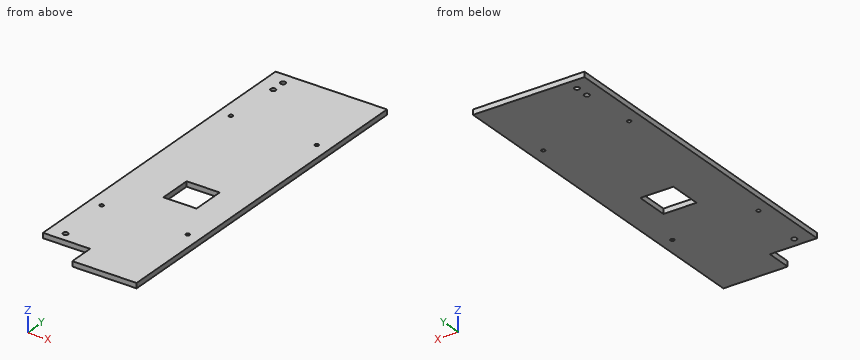
from build123d import *

# Parameters (mm, degrees)
ESQUISSE1_R      = 1.5
ESQUISSE1_R_2    = 2
ESQUISSE1_W      = 26
ESQUISSE1_H      = 26
EXTRUSION1_DEPTH = 4


with BuildPart() as part:
    # Esquisse1 → Extrusion1 (new body)
    with BuildSketch(Plane.XY):
        Polygon((-30.537686248, 34.180421053), (56.962313752, 34.180421053), (56.962313752, -246.819578947), (6.462313752, -246.819578947), (6.462313752, -226.819578947), (-30.537686248, -226.819578947), align=None)
        with Locations((-20.537686248, -175.319578947)):
            Circle(ESQUISSE1_R, mode=Mode.SUBTRACT)
        with Locations((-20.537686248, -30.319578947)):
            Circle(ESQUISSE1_R, mode=Mode.SUBTRACT)
        with Locations((46.962313752, -30.319578947)):
            Circle(ESQUISSE1_R, mode=Mode.SUBTRACT)
        with Locations((46.962313752, -175.319578947)):
            Circle(ESQUISSE1_R, mode=Mode.SUBTRACT)
        with Locations((-18.037686248, -219.319578947)):
            Circle(ESQUISSE1_R_2, mode=Mode.SUBTRACT)
        with Locations((-18.037686248, 24.680421053)):
            Circle(ESQUISSE1_R_2, mode=Mode.SUBTRACT)
        with Locations((-18.037686248, 13.680421053)):
            Circle(ESQUISSE1_R_2, mode=Mode.SUBTRACT)
        with Locations((18.962313752, -130.819578947)):
            Rectangle(ESQUISSE1_W, ESQUISSE1_H, mode=Mode.SUBTRACT)
    extrude(amount=EXTRUSION1_DEPTH)


solid = part.part
Could you check a few things on this model? Use its own coordinates, in mm. Give positions to 0.01 mm unless a question says otherwise; leave off trailing zeros. Order: outer loops, then holes, each group sorted by start corner. A loop starts at its lowest first (then second) coordinate and runs counter-clockwise, first axis right, second up. Notation, with made-up numbers: (-16, -9.75) - (23, -9.75) arc R18 ccw to (23, 19.25) - close; hole circle Ø2 at (-33, 47.25). An arc over 180 degrees is marked (long way). One line per question, with ' | ' between items. Start each with the question number.
Item 1: I want a section at A-A on y = -124. Write out the boundary of the cut face in (x, z).
Item 2: I need wall thicknesses on probe 1 along Y at (x, z) = (26, 2.55); probe 2 along Y at (x, z) = (2.5, 0.5); probe 3 along X at (y, z) = (-229, 2.6). Which ranges of each line are inside material? Lowest first, please. Write a range as [from, to].
Item 3: I want a section at B-B on x = 22. Write out the boundary of the cut face in (y, z).
Item 4: I'm going to push flat-ended pins straight in: pin 1 Ø3 at (x, y) = (-18.04, -219.32) entering from +Z; pin 2 Ø1.2 at (x, z) = (-8, 3) entering from -Y. Where does each tip first touch, or does it pass through?
Item 5: I want a section at D-D on x = -7. Write out the boundary of the cut face in (y, z), then the cut area to 3 significant figures.
Item 6: I want a section at C-C on z = 1.85. Give the number of separate pieces and of enclosed holes in the cut face, then the cut area to 3 significant figures.
Verdict:
1) outline: (-30.54, 0) - (5.96, 0) - (5.96, 4) - (-30.54, 4) - close; (31.96, 0) - (56.96, 0) - (56.96, 4) - (31.96, 4) - close
2) probe 1: [-246.82, -143.82], [-117.82, 34.18] | probe 2: [-226.82, 34.18] | probe 3: [6.46, 56.96]
3) outline: (-246.82, 0) - (-143.82, 0) - (-143.82, 4) - (-246.82, 4) - close; (-117.82, 0) - (34.18, 0) - (34.18, 4) - (-117.82, 4) - close
4) pin 1: through | pin 2: y = -226.82
5) outline: (-226.82, 0) - (34.18, 0) - (34.18, 4) - (-226.82, 4) - close | area: 1,040 mm^2
6) separate pieces: 1 | enclosed holes: 8 | area: 23,100 mm^2
